Model file for the job. Use its own axes, mm. Face numbers are marked on the shaded views. A direction names the side the tool comes from. Give positions to 0.01 mm unless a question says otherwise; leave off trailing zeros. Order: outer loops, then holes, each group sorted by start corner. A loop starts at its lowest first (then second) coordinate and runs counter-clockwise, first axis right, second up. Notation, with made-up numbers: (-24.75, -0.5) -> (-1.75, -0.5) arc R23 cw to (-1.75, 13.5) -> close; hole circle Ø1 at (-15, 30). An arc over 180 degrees is marked (long way). Use CSV: the item, a comma, the result in double quotes. Start each with the question number.
1. Wall check: line 1 (Y direction, x = 24, z = 15.25); line 2 (Z direction, x = 32, y = 26); line 3 (X direction, y = 31.5, z = 23). Give the ranges that are in metal, low to high. Write a range as from..to.
2. 3-axis set-ups, long thin cutter, end or side, ignore diameter. For the marked faces 1 and 2: which of +Z, -Z, +X, -X, +Y, -Y reach the whole face in a straight line?
3. Pull direction Y, two halves, no side cores. Call the marked faces 3, 4, 5 and 6: released by +Y, released by -Y, zero draft, split by the parting line, or undercut.
4. Drop flat-ended pins along their axis: pin 1 (1 mm diameter, centred on y = 41, z = 3, fed in from +X); pin 2 (12 mm diameter, centred on x = 21.5, y = 37.5, fed in from +Z). Give the stop position or say it passes through.
5. Cut at C-C on y = 43. List the corners of the cut face in (x, z) (1 decimal), then the cut area to 3 significant figures.
```python
from build123d import *

# Parameters (mm, degrees)
F1_DEPTH = 25.4
F3_DEPTH = 1.5875
F4_SIZE  = 0.635


with BuildPart() as f1:
    # F0 (on Top) → F1 (new body)
    with BuildSketch(Plane.XY):
        with BuildLine():
            Line((38.1, 0), (12.7, 0))
            ThreePointArc((12.7, 0), (3.719744, 3.719744), (0, 12.7))
            Line((0, 12.7), (0, 44.45))
            ThreePointArc((0, 44.45), (3.719744, 53.430256), (12.7, 57.15))
            Line((12.7, 57.15), (38.1, 57.15))
            Line((38.1, 57.15), (38.1, 58.7375))
            Line((38.1, 58.7375), (12.7, 58.7375))
            ThreePointArc((12.7, 58.7375), (2.597212, 54.552788), (-1.5875, 44.45))
            Line((-1.5875, 44.45), (-1.5875, 12.7))
            ThreePointArc((-1.5875, 12.7), (2.597212, 2.597212), (12.7, -1.5875))
            Line((12.7, -1.5875), (38.1, -1.5875))
            Line((38.1, -1.5875), (38.1, 0))
        make_face()
    extrude(amount=F1_DEPTH)

    # F2 (on face) → F3 (join)
    with BuildSketch(Plane(origin=(0, 0, 0), x_dir=(1, 0, 0), z_dir=(0, 0, -1))):
        with BuildLine():
            Line((38.1, 0), (12.7, 0))
            ThreePointArc((12.7, 0), (3.719744, -3.719744), (0, -12.7))
            Line((0, -12.7), (0, -44.45))
            ThreePointArc((0, -44.45), (3.719744, -53.430256), (12.7, -57.15))
            Line((12.7, -57.15), (38.1, -57.15))
            Line((38.1, -57.15), (38.1, 0))
        make_face()
    extrude(amount=-F3_DEPTH)

    # F4
    f4_edges = [f1.edges().sort_by_distance(p)[0] for p in [
        (25.4, -1.5875, 0),
        (38.1, 28.575, 0),
        (25.4, 58.7375, 0),
        (2.597212, 54.552788, 0),
        (-1.5875, 28.575, 0),
        (2.597212, 2.597212, 0),
    ]]
    chamfer(f4_edges, length=F4_SIZE)


solid = f1.part
```
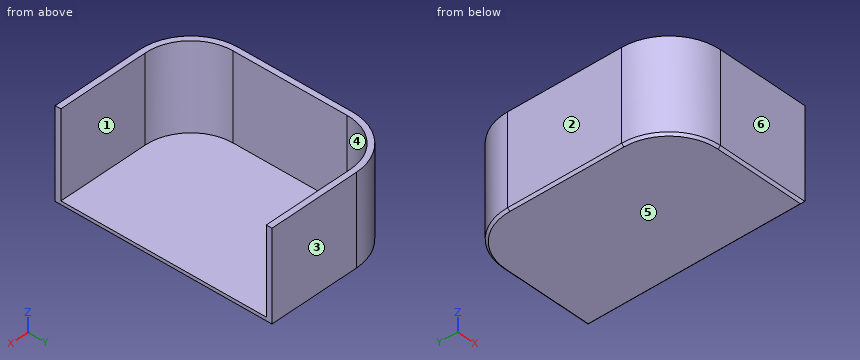
Verdict:
1,line 1,"-1.59..0, 57.15..58.74"
1,line 2,"0..1.59"
1,line 3,"-1.59..0"
2,face 1,"+Z, +X"
2,face 2,"+Z, -Z, -X, +Y, -Y"
3,face 3,"released by +Y"
3,face 4,"undercut"
3,face 5,"zero draft"
3,face 6,"released by -Y"
4,pin 1,"x = 0"
4,pin 2,"z = 1.59"
5,outline,"(-1.6, 0.6) -> (-1, 0) -> (37.5, 0) -> (38.1, 0.6) -> (38.1, 1.6) -> (0, 1.6) -> (0, 25.4) -> (-1.6, 25.4) -> close"
5,area,"100 mm^2"
